Verification items for the finished model (mm, model axes). A direction names the side the tool comes from. Give positions to 0.01 mm unless a question says otherwise; leave off trailing zeros. Write each loop counter-clockwise with the first axis right and the second up, starting at its lowest first coordinate (ties: lowest second). Pieces come first, ordered by that corner, then holes. Notation, with made-up numbers: (-39.75, -18.75) -> (-8.75, -18.75) arc R24 cw to (-8.75, 3.25) -> close; hole circle Ø11 at (44.25, 60). An arc over 180 degrees is marked (long way). Use one line per item in the form item = value. Start each with the question number.
(1) Section check B-B, the plane y = 115.57. Record the cut outline in (x, z) (3 decimals).
(2) Set-up check for faces 1 (the face through (29.58, 93.59, 3.26)), 2 (the face through (39, 123.825, 15)), 3 (the face through (1.565, 37.594, 23.88)): record each of +Z, -Z, +X, -X, +Y, -Y from which the full face is reachable in a straight line by a thin tool's end or side.
(3) Section check A-A, the plane x = 60.96. Record the cut outline in (y, z) (3 decimals), plus the area to 3 significant figures.
(4) Section check C-C, the plane z = 11.75. Record the cut outline in (x, y) (3 decimals).
(5) Scan lines: L1, parallel to Y at x = 60.96, z = 3.5; L2, parallel to Y at x = 21.59, z = 4.5; L3, parallel to Y at x = 8.89, z = 4.25. Record each from-to range of solid material in increasing order.
(6) Depth check by flat-ended pin: pin 1 Ø3 at (x, y) = (67.31, 53.34) entering from -Z; pin 2 Ø3 at (x, y) = (34.5, 48.5) entering from +Z. Enter the tip coordinate at first touch or a pass-through.
(7) Section check D-D, the plane y = 33.02. Record the cut outline in (x, z).
from build123d import *

# Parameters (mm, degrees)
SKETCH1_W           = 127
SKETCH1_H           = 76.2
BOSS_EXTRUDE1_DEPTH = 6.604
HOLE2_D             = 3.4
HOLE2_DEPTH         = 7
HOLE3_D             = 4
HOLE3_DEPTH         = 7
BOSS_EXTRUDE2_DEPTH = 18
FILLET1_R           = 2.54


with BuildPart() as part:
    # Sketch1 → Boss-Extrude1 (new body)
    with BuildSketch(Plane(origin=(0, 0, 0), x_dir=(0, 1, 0), z_dir=(0, 0, 1))):
        with Locations((63.5, -38.1)):
            Rectangle(SKETCH1_W, SKETCH1_H)
    extrude(amount=BOSS_EXTRUDE1_DEPTH)

    # Hole2
    with Locations(Plane.XY.offset(6.604)):
        with Locations((54.61, 73.66), (15.24, 15.24), (60.96, 15.24), (60.96, 33.02), (15.24, 33.02), (8.89, 53.34), (21.59, 53.34), (21.59, 73.66), (8.89, 73.66), (8.89, 95.25), (29.21, 95.25), (29.21, 115.57), (8.89, 115.57), (54.61, 53.34), (67.31, 53.34), (67.31, 73.66)):
            Hole(HOLE2_D / 2, depth=HOLE2_DEPTH)

    # Hole3
    with Locations(Plane.XY.offset(6.604)):
        with Locations((67.31, 115.57), (54.61, 115.57), (54.61, 95.25), (67.31, 95.25)):
            Hole(HOLE3_D / 2, depth=HOLE3_DEPTH)

    # Sketch12 → Boss-Extrude2 (add)
    with BuildSketch(Plane.XY.offset(6.604)):
        Polygon((3.175, 123.825), (3.175, 36.83), (0, 36.83), (0, 127), (76.2, 127), (76.2, 36.83), (73.025, 36.83), (73.025, 123.825), align=None)
        Polygon((0, 0), (76.2, 0), (76.2, 11.43), (73.025, 11.43), (73.025, 3.175), (3.175, 3.175), (3.175, 11.43), (0, 11.43), align=None)
    extrude(amount=BOSS_EXTRUDE2_DEPTH)

    # Fillet1
    fillet1_edges = [part.edges().sort_by_distance(p)[0] for p in [
        (1.5875, 36.83, 24.604),
        (74.6125, 36.83, 24.604),
        (74.6125, 11.43, 24.604),
        (1.5875, 11.43, 24.604),
    ]]
    fillet(fillet1_edges, radius=FILLET1_R)


solid = part.part
Completed:
q1.outline = (0, 0) -> (7.19, 0) -> (7.19, 6.604) -> (3.175, 6.604) -> (3.175, 24.604) -> (0, 24.604) -> close; (10.59, 0) -> (27.51, 0) -> (27.51, 6.604) -> (10.59, 6.604) -> close; (30.91, 0) -> (52.61, 0) -> (52.61, 6.604) -> (30.91, 6.604) -> close; (56.61, 0) -> (65.31, 0) -> (65.31, 6.604) -> (56.61, 6.604) -> close; (69.31, 0) -> (76.2, 0) -> (76.2, 24.604) -> (73.025, 24.604) -> (73.025, 6.604) -> (69.31, 6.604) -> close
q2.face_1 = +Z, -Z
q2.face_2 = +Z
q2.face_3 = +Z, +X, -X
q3.outline = (0, 0) -> (13.54, 0) -> (13.54, 6.604) -> (3.175, 6.604) -> (3.175, 24.604) -> (0, 24.604) -> close; (16.94, 0) -> (31.32, 0) -> (31.32, 6.604) -> (16.94, 6.604) -> close; (34.72, 0) -> (127, 0) -> (127, 24.604) -> (123.825, 24.604) -> (123.825, 6.604) -> (34.72, 6.604) -> close
q3.area = 908 mm²
q4.outline = (0, 0) -> (76.2, 0) -> (76.2, 11.43) -> (73.025, 11.43) -> (73.025, 3.175) -> (3.175, 3.175) -> (3.175, 11.43) -> (0, 11.43) -> close; (0, 36.83) -> (3.175, 36.83) -> (3.175, 123.825) -> (73.025, 123.825) -> (73.025, 36.83) -> (76.2, 36.83) -> (76.2, 127) -> (0, 127) -> close
q5.L1 = 0 to 13.54, 16.94 to 31.32, 34.72 to 127
q5.L2 = 0 to 51.64, 55.04 to 71.96, 75.36 to 127
q5.L3 = 0 to 51.64, 55.04 to 71.96, 75.36 to 93.55, 96.95 to 113.87, 117.27 to 127
q6.pin_1 = through
q6.pin_2 = 6.6
q7.outline = (0, 0) -> (13.54, 0) -> (13.54, 6.6) -> (0, 6.6) -> close; (16.94, 0) -> (59.26, 0) -> (59.26, 6.6) -> (16.94, 6.6) -> close; (62.66, 0) -> (76.2, 0) -> (76.2, 6.6) -> (62.66, 6.6) -> close
